For this review, take the finished solid that the model builds, in its own axes (mm). A direction names the side the tool comes from. Give positions to 0.01 mm unless a question says otherwise; leave off trailing zeros. Loops run counter-clockwise (first coordinate to the right, second up) from the corner with the lowest first, then second, coordinate; pieces in that order, holes last.
```python
from build123d import *

# Parameters (mm, degrees)
BODY_START         = 12
SKETCH1_W          = 40
SKETCH1_H          = 35
BODY_DEPTH         = 26
PORT_IN_G12_START  = -30
SKETCH2_R          = 10.45
PORT_IN_G12_DEPTH  = 10
PORT_OUT_G12_START = 20
SKETCH3_R          = 10.45
PORT_OUT_G12_DEPTH = 10
SKETCH4_W          = 24
SKETCH4_H          = 21
FEET_DEPTH         = 12
FLOW_ARROW_START   = 38
FLOW_ARROW_DEPTH   = 0.8
WIRE_EXIT_START    = 38
SKETCH6_W          = 6
SKETCH6_H          = 10
WIRE_EXIT_DEPTH    = 3


with BuildPart() as part:
    # Sketch1 → Body (new body)
    with BuildSketch(Plane(origin=(0, 0, 0), x_dir=(1, 0, 0), z_dir=(0, 1, 0)).offset(BODY_START)):
        Rectangle(SKETCH1_W, SKETCH1_H)
    extrude(amount=BODY_DEPTH)

    # Sketch2 → Port_In_G12 (add)
    with BuildSketch(Plane(origin=(0, 0, 0), x_dir=(0, 0, -1), z_dir=(1, 0, 0)).offset(PORT_IN_G12_START)):
        with Locations((0, 25)):
            Circle(SKETCH2_R)
    extrude(amount=PORT_IN_G12_DEPTH)

    # Sketch3 → Port_Out_G12 (add)
    with BuildSketch(Plane(origin=(0, 0, 0), x_dir=(0, 0, -1), z_dir=(1, 0, 0)).offset(PORT_OUT_G12_START)):
        with Locations((0, 25)):
            Circle(SKETCH3_R)
    extrude(amount=PORT_OUT_G12_DEPTH)

    # Sketch4 → Feet (add)
    with BuildSketch(Plane(origin=(0, 0, 0), x_dir=(1, 0, 0), z_dir=(0, 1, 0))):
        Rectangle(SKETCH4_W, SKETCH4_H)
    extrude(amount=FEET_DEPTH)

    # Sketch5 → Flow_Arrow (add)
    with BuildSketch(Plane(origin=(0, 0, 0), x_dir=(1, 0, 0), z_dir=(0, 1, 0)).offset(FLOW_ARROW_START)):
        Polygon((-12, 3), (4, 3), (4, 7), (13, 0), (4, -7), (4, -3), (-12, -3), align=None)
    extrude(amount=FLOW_ARROW_DEPTH)

    # Sketch6 → Wire_Exit (add)
    with BuildSketch(Plane(origin=(0, 0, 0), x_dir=(1, 0, 0), z_dir=(0, 1, 0)).offset(WIRE_EXIT_START)):
        with Locations((-14, 0)):
            Rectangle(SKETCH6_W, SKETCH6_H)
    extrude(amount=WIRE_EXIT_DEPTH)


solid = part.part
```
Q1. Consider section A-A on y = 25. Give the boundary of the cut face in (x, z).
Answers:
outline: (-30, -10.45) - (-20, -10.45) - (-20, -17.5) - (20, -17.5) - (20, -10.45) - (30, -10.45) - (30, 10.45) - (20, 10.45) - (20, 17.5) - (-20, 17.5) - (-20, 10.45) - (-30, 10.45) - close
Q2. For probe 1 along Y at (x, z) = (12.5, 4.5); probe 2 along Y at (x, z) = (5, -4); probe 3 along X at (y, z) = (37, -1.5), list the stretches that pass through material, from the lowest coordinate up.
Answers:
probe 1: y = 12 to 38
probe 2: y = 0 to 38.8
probe 3: x = -20 to 20
Q3. Consider section C-C on z = -13. Give the boundary of the cut face in (x, y), plus the area to 3 significant figures.
Answers:
outline: (-20, 12) - (20, 12) - (20, 38) - (-20, 38) - close
area: 1,040 mm2
Q4. Machinability: for faces 1 (the flat face through (0, 6, -10.5)), 2 (the flat face through (-20, 13, 0)), 3 (the flat face through (-14, 39, -5)), 4 (the flat face through (8.563, 38.394, 3.451)), 5 (the cylindrical face through (24.93, 33.81, -5.62)), which of the approach directions +Z, -Z, +X, -X, +Y, -Y give a long, thin tool a straight path to every point of the face, cutting with its end or side? Answer none if there is none.
Answers:
face 1: -Z, +X, -X, -Y
face 2: -X
face 3: -Z, -X, +Y
face 4: +Z, +X, +Y
face 5: +X
Q5. For pin 1 Ø10.5 at (x, z) = (8, 0.5) entering from +Y; pin 2 Ø3.5 at (y, z) = (7.5, 1) entering from +X; pin 3 Ø1 at (x, z) = (-16, 10.5) entering from +Y, all flat-tipped, find the tip position at first contact; note any pin that passes through.
Answers:
pin 1: stops at y = 38.8
pin 2: stops at x = 12
pin 3: stops at y = 38
Q6. Consider section B-B on x = -19. Give the boundary of the cut face in (y, z), plus the area to 3 significant figures.
Answers:
outline: (12, -17.5) - (38, -17.5) - (38, 17.5) - (12, 17.5) - close
area: 910 mm2
Q7. Consider section D-D on y = 16.5. Give the boundary of the cut face in (x, z).
Answers:
outline: (-30, -6.08) - (-20, -6.08) - (-20, -17.5) - (20, -17.5) - (20, -6.08) - (30, -6.08) - (30, 6.08) - (20, 6.08) - (20, 17.5) - (-20, 17.5) - (-20, 6.08) - (-30, 6.08) - close
